from build123d import *

# Parameters (mm, degrees)
SKETCH_1_W      = 300
SKETCH_1_H      = 20
SKETCH_1_R      = 7
EXTRUDE_1_DEPTH = 10
FILLET_1_R      = 10


with BuildPart() as part:
    # 草图1 → 凸台-拉伸1 (new body)
    with BuildSketch(Plane.XY):
        Rectangle(SKETCH_1_W, SKETCH_1_H)
        with Locations((-140, 0)):
            Circle(SKETCH_1_R, mode=Mode.SUBTRACT)
        with Locations((140, 0)):
            Circle(SKETCH_1_R, mode=Mode.SUBTRACT)
    extrude(amount=EXTRUDE_1_DEPTH)

    # 圆角1
    fillet_1_edges = [part.edges().sort_by_distance(p)[0] for p in [
        (150, 10, 5),
        (150, -10, 5),
        (-150, -10, 5),
        (-150, 10, 5),
    ]]
    fillet(fillet_1_edges, radius=FILLET_1_R - 0.0001)  # a hair under: the kernel refuses the full size


solid = part.part
Source: CAD feature listing. Evaluate the final solid. Frame: model axes, mm. Coordinates: 2 decimals unless noted, no trailing zeros.
Item 1: Cut plane A-A (z = 5.75). Count the separate pieces of the cut face and the enclosed holes in it, plus the area to 3 significant figures.
Output values:
separate pieces: 1
enclosed holes: 2
area: 5,610 mm2
Item 2: Material intervals for line 1 (X direction, y = -0.25, z = 1.5); line 2 (Y direction, x = 140, z = 3.75); line 3 (X direction, y = -2, z = 5.25), sorted ascending.
Output values:
line 1: x = -150 to -147, -133 to 133, 147 to 150
line 2: y = -10 to -7, 7 to 10
line 3: x = -149.8 to -146.71, -133.29 to 133.29, 146.71 to 149.8
Item 3: First-contact query: P1, Ø8.5, axis at x = -140, y = 0, coming from the +Z side; P2, Ø1.5, axis at y = -4.5, z = 3.5, coming from the -X side; P3, Ø2, axis at x = 7.5, y = 3.5, coming from the -Z side; P4, Ø3, axis at y = 4, z = 2.5, coming from the -X side. Flat tips, straight axial feed; report the tip coordinate or a pass-through.
Output values:
P1: passes through
P2: stops at x = -149.27
P3: stops at z = 0
P4: stops at x = -149.68
Item 4: Pull-direction query (X, two-part tool) for faces 1 (the face through (-147.15, 6.99, 5.07)), 2 (the face through (-145.16, 4.73, 4.93)), 3 (the face through (-2, 10, 5)); classes: pulls with the +X half, pulls with the -X half, needs draft (parallel to the pull), parting line crosses it, or undercut.
Output values:
face 1: pulls with the -X half
face 2: undercut
face 3: needs draft
